Part print with two shaded views. Sizes in mm from the minimum x, y, z corner. A direction names the side the tool comes from. Give positions to 0.01 mm unless a question says otherwise; leave off trailing zeros. Order: outer loops, then holes, each group sorted by start corner. A loop starts at its lowest first (then second) coordinate and runs counter-clockwise, first axis right, second up. Notation, with made-up numbers: M 10,14.25 L 62,14.25 A18 ccw 62,47.25 Z; hole C -9.5,-26.5 d5. An arc over 180 degrees is marked long. Answer as CSV lines item,"result".
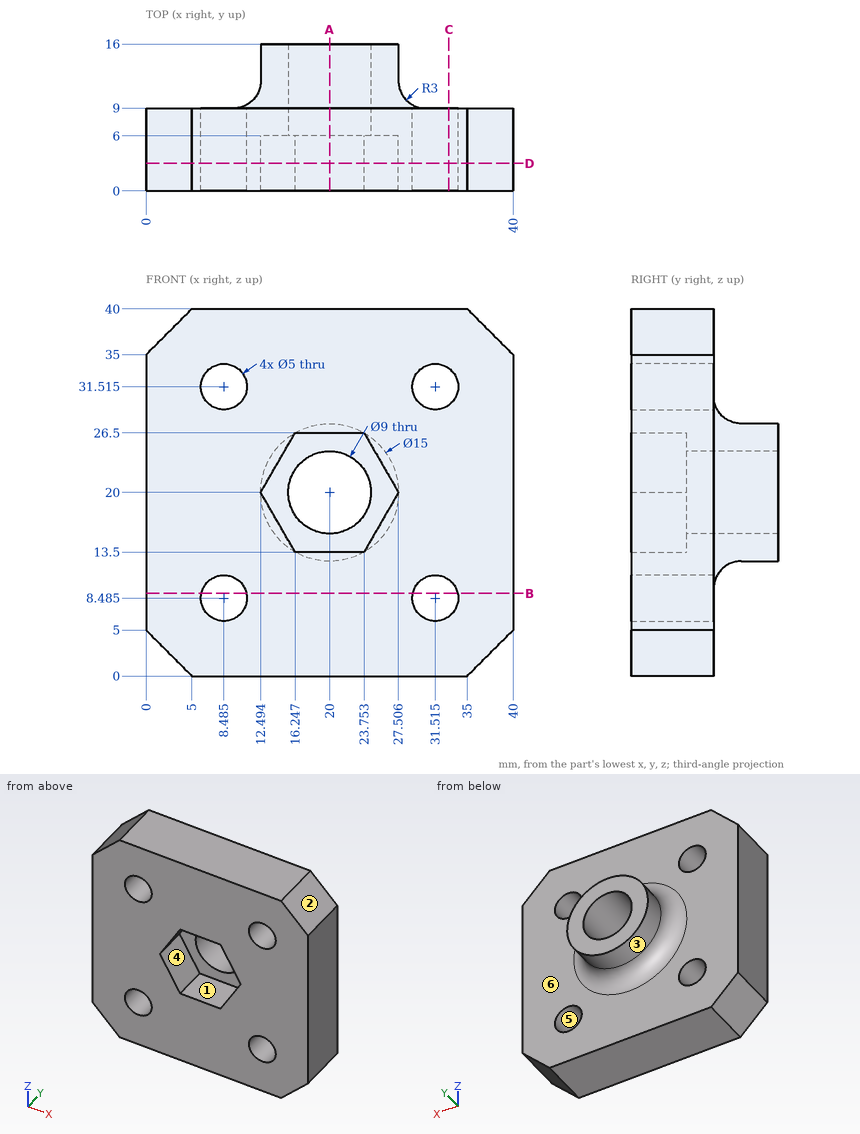
Item 1: Probe line 1 along X through (y, z) = (1.5, 31.5) (1 decimal); line 2 along Z through (x, y) = (17, 1.75); line 3 along X through (y, z) = (3.5, 10.5) (1 decimal). List the from-to ranges inside material, lowest first. Write a range as from..to.
Geometry says:
line 1,"x = 0..6, 11..29, 34..40"
line 2,"z = 0..13.5, 26.5..40"
line 3,"x = 0..7, 10..30, 33..40"
Item 2: Band-saw the part on C-C (x = 33). Give the cut face in (y, z) (1 decimal).
Geometry says:
outline,"M 0,0 L 9,0 L 9,6.5 L 0,6.5 Z; M 0,10.5 L 9,10.5 L 9,29.5 L 0,29.5 Z; M 0,33.5 L 9,33.5 L 9,40 L 0,40 Z"
Item 3: Drop flat-ended pins along their axis: pin 1 (12 mm diameter, centred on x = 34.5, z = 8, fed in from +Y); pin 2 (6.5 mm diameter, centred on x = 19, z = 19.5, fed in from -Y); pin 3 (4 mm diameter, centred on x = 11.5, y = 14, fed in from +Z). Give the stop position or say it passes through.
Geometry says:
pin 1,"stops at y = 9"
pin 2,"passes through"
pin 3,"stops at z = 23.74"
Item 4: 3-axis set-ups, long thin cutter, end or side, ignore diameter. For the marked faces 1 and 2: which of +Z, -Z, +X, -X, +Y, -Y reach the whole face in a straight line?
Geometry says:
face 1,"-Y"
face 2,"+Z, +X, +Y, -Y"
Item 5: Band-saw the part on B-B (z = 9). Give the cut face in (x, y), and give its area (3 significant figures).
Geometry says:
outline,"M 0,0 L 6.04,0 L 6.04,9 L 0,9 Z; M 10.93,0 L 29.07,0 L 29.07,9 L 10.93,9 Z; M 33.96,0 L 40,0 L 40,9 L 33.96,9 Z"
area,"272 mm2"
Item 6: Band-saw the part on D-D (y = 3). Give the cut face in (x, z) (1 decimal).
Geometry says:
outline,"M 0,5 L 5,0 L 35,0 L 40,5 L 40,35 L 35,40 L 5,40 L 0,35 Z; hole C 8.5,8.5 d5; hole C 8.5,31.5 d5; hole M 12.5,20 L 16.2,13.5 L 23.8,13.5 L 27.5,20 L 23.8,26.5 L 16.2,26.5 Z; hole C 31.5,8.5 d5; hole C 31.5,31.5 d5"
Item 7: Band-saw the part on A-A (x = 20). Give the cut face in (y, z).
Geometry says:
outline,"M 0,0 L 9,0 L 9,9.5 A3 cw 12,12.5 L 16,12.5 L 16,15.5 L 6,15.5 L 6,13.5 L 0,13.5 Z; M 0,26.5 L 6,26.5 L 6,24.5 L 16,24.5 L 16,27.5 L 12,27.5 A3 cw 9,30.5 L 9,40 L 0,40 Z"
Item 8: Pull direction X, two halves, no side cores. Call the marked faces 3, 4, 5 and 6: released by +X, released by -X, zero draft, split by the parting line, or undercut.
Geometry says:
face 3,"split by the parting line"
face 4,"undercut"
face 5,"undercut"
face 6,"zero draft"
